Geometry check sheet. Reference: the model listing, model coordinates, mm. Coordinates: 2 decimals unless noted, no trailing zeros. Write each loop counter-clockwise with the first axis right and the second up, starting at its lowest first coordinate (ties: lowest second). Pieces come first, ordered by that corner, then holes. Notation, with made-up numbers: (7, 68.25) -> (28, 68.25) arc R14 cw to (28, 80.25) -> close; hole circle Ø9 at (68.25, -24). An arc over 180 degrees is marked (long way). Answer as CSV lines item,"result".
```python
from build123d import *

# Parameters (mm, degrees)
TD_SKETCH_R                             = 0.79248
TL_FEATURE_DEPTH                        = 21.0312
TDF_STD_SKETCH_W                        = 2.09296
TDF_STD_SKETCH_H                        = 2.09296
TDF_STD_FEATURE_DEPTH                   = 22.061040395
ISA_20_STD_FEATURE_DEPTH                = 22.061040395
ISA_20_STD_FEATURE_DEPTH_BACK           = 22.061040395
F_10BA_STD_FEATURE_DEPTH                = 22.061040395
F_10BA_STD_FEATURE_DEPTH_BACK           = 22.061040395
FRO_STD_FEATURE_DEPTH                   = 22.061040395
FRO_STD_FEATURE_DEPTH_BACK              = 22.061040395
C_STD_FEATURE_DEPTH                     = 22.061040395
C_STD_FEATURE_DEPTH_BACK                = 22.061040395
ERW_STD_FEATURE_DEPTH                   = 0.01905
H_STD_FEATURE_REACH                     = 22.955
H_STD_SKETCH_R                          = 0.01905
H_STD_SKETCH_3_R                        = 0.01905
FUNNEL_FINAL_DIAMETRE_STD_FEATURE_DEPTH = 2.499995
FUNNEL_FINAL_DIAMETRE_STD_FEATURE_DRAFT = -22.5
ROUND_BR_STD_FEATURE_START              = -1
ROUND_BR_STD_FEATURE_DEPTH              = 0.939082249


with BuildPart() as part:
    # TD_sketch → TL_feature (new body)
    with BuildSketch(Plane(origin=(0, 0, 0), x_dir=(1, 0, 0), z_dir=(0, 1, 0))):
        with Locations(Location((0, 0, 0), (0, 0, 270))):
            Circle(TD_SKETCH_R)
    extrude(amount=TL_FEATURE_DEPTH)

    # TDF_STD_sketch → TDF_STD_feature (cut, through all)
    with BuildSketch(Plane(origin=(0, 0, 0), x_dir=(1, 0, 0), z_dir=(0, 1, 0))):
        with Locations((-1.4224, 0)):
            Rectangle(TDF_STD_SKETCH_W, TDF_STD_SKETCH_H)
    extrude(amount=TDF_STD_FEATURE_DEPTH, mode=Mode.SUBTRACT)

    # ISA_20_STD_sketch → ISA_20_STD_feature (cut, two sides: drawn at the far end of the back side and taken through both)
    with BuildSketch(Plane(origin=(0, 0, 0), x_dir=(0, 0, -1), z_dir=(1, 0, 0)).offset(-ISA_20_STD_FEATURE_DEPTH_BACK)):
        Polygon((-12.955177728, 73.256388083), (-3.746467997, 21.0312), (-0.0381, 0), (0.0381, 0), (3.746467997, 21.0312), (12.955177728, 73.256388083), (12.955177728, -32.805303497), (-12.955177728, -32.805303497), align=None)
    extrude(amount=ISA_20_STD_FEATURE_DEPTH + ISA_20_STD_FEATURE_DEPTH_BACK, mode=Mode.SUBTRACT)

    # 10BA_STD_sketch → 10BA_STD_feature (cut, two sides: drawn at the far end of the back side and taken through both)
    with BuildSketch(Plane.XY.offset(-F_10BA_STD_FEATURE_DEPTH_BACK)):
        Polygon((-53.187771959, 0), (-0.37592, 0), (-0.29972, 0), (-0.091356515, 0.029283578), (3.611847997, 21.0312), (12.782529849, 73.04072126), (91.167207296, 2.243763904), (25.196905488, -70.796957355), align=None)
    extrude(amount=F_10BA_STD_FEATURE_DEPTH + F_10BA_STD_FEATURE_DEPTH_BACK, mode=Mode.SUBTRACT)

    # FRO_STD_sketch → FRO_STD_feature (cut, two sides: drawn at the far end of the back side and taken through both)
    with BuildSketch(Plane.XY.offset(-FRO_STD_FEATURE_DEPTH_BACK)):
        with BuildLine():
            Line((-0.37592, 52.149873762), (-0.37592, 0.0254))
            ThreePointArc((-0.37592, 0.0254), (-0.368480512, 0.007439488), (-0.35052, 0))
            Line((-0.35052, 0), (51.773953762, 0))
            Line((51.773953762, 0), (-21.941183964, -73.715137726))
            Line((-21.941183964, -73.715137726), (-74.091057726, -21.565263964))
            Line((-74.091057726, -21.565263964), (-0.37592, 52.149873762))
        make_face()
    extrude(amount=FRO_STD_FEATURE_DEPTH + FRO_STD_FEATURE_DEPTH_BACK, mode=Mode.SUBTRACT)

    # C_STD_sketch → C_STD_feature (cut, two sides: drawn at the far end of the back side and taken through both)
    with BuildSketch(Plane(origin=(0, 0, 0), x_dir=(0, 0, -1), z_dir=(1, 0, 0)).offset(-C_STD_FEATURE_DEPTH_BACK)):
        with BuildLine():
            Line((-51.36762506, -8.882670253), (-0.03551364, 0))
            ThreePointArc((-0.03551364, 0), (0, 0.003050032), (0.03551364, 0))
            Line((0.03551364, 0), (51.36762506, -8.882670253))
            Line((51.36762506, -8.882670253), (51.36762506, -113.072640858))
            Line((51.36762506, -113.072640858), (-51.36762506, -113.072640858))
            Line((-51.36762506, -113.072640858), (-51.36762506, -8.882670253))
        make_face()
    extrude(amount=C_STD_FEATURE_DEPTH + C_STD_FEATURE_DEPTH_BACK, mode=Mode.SUBTRACT)


with BuildPart() as body_2:
    # ERW_STD_sketch → ERW_STD_feature (new, symmetric)
    with BuildSketch(Plane.XY):
        Polygon((-0.182120032, 0.06096), (-0.182120032, 0), (-0.321820032, 0), (-0.275883377, 0.06096), align=None)
    extrude(amount=ERW_STD_FEATURE_DEPTH, both=True)

    # H_STD_sketch → H_STD_feature (add, up to next)
    with BuildSketch(Plane(origin=(-0.096909952, 0.110156063, 0), x_dir=(0, 0, -1), z_dir=(0.8660254037844415, 0.4999999999999953, 0)), mode=Mode.PRIVATE) as h_std_feature_sk1:
        with Locations(Location((0, 0, 0), (0, 0, 90))):
            Circle(H_STD_SKETCH_R)
    h_std_feature_tool1 = extrude(h_std_feature_sk1.sketch, amount=-H_STD_FEATURE_REACH, mode=Mode.PRIVATE) - body_2.part
    add(h_std_feature_tool1.solids().sort_by_distance((-0.09691, 0.110156, 0))[0])


with BuildPart() as funnel_final_diametre_std_feature_tool:
    # H_STD_sketch<3> → funnel_final_diametre_STD_feature (with draft: the straight prism first)
    with BuildSketch(Plane(origin=(-0.096909952, 0.110156063, 0), x_dir=(0, 0, -1), z_dir=(0.8660254037844415, 0.4999999999999953, 0))):
        with Locations(Location((0, 0, 0), (0, 0, 90))):
            Circle(H_STD_SKETCH_3_R)
    extrude(amount=FUNNEL_FINAL_DIAMETRE_STD_FEATURE_DEPTH)
    # funnel_final_diametre_STD_feature: the draft: its side faces are tilted about the plane it starts from
    funnel_final_diametre_std_feature_sides = [funnel_final_diametre_std_feature_tool.faces().sort_by_distance(p)[0] for p in [
        (0.995144638, 0.718657029, 0),
    ]]
    draft(funnel_final_diametre_std_feature_sides, Plane(origin=(-0.096909952, 0.110156063, 0), x_dir=(0, 0, -1), z_dir=(0.8660254037844415, 0.4999999999999953, 0)), FUNNEL_FINAL_DIAMETRE_STD_FEATURE_DRAFT)


with BuildPart() as body_2_1:
    add(body_2.part)

    # funnel_final_diametre_STD_feature: add funnel_final_diametre_std_feature_tool
    add(funnel_final_diametre_std_feature_tool.part)

    # ROUND_BR_STD_feature: read off the stored shape, not the designer's step
    # ROUND_BR_STD_feature outline → ROUND_BR_STD_feature (cut)
    with BuildSketch(Plane(origin=(0, 0, 0), x_dir=(0.79863551004729, -0.601815023152052, 0), z_dir=(0.601815023152052, 0.79863551004729, 0)).offset(ROUND_BR_STD_FEATURE_START)):
        with BuildLine():
            Line((-0.257016905, -0.01905), (-0.237966905, -0.01905))
            ThreePointArc((-0.237966905, -0.01905), (-0.251437289, -0.013470384), (-0.257016905, 0))
            Line((-0.257016905, 0), (-0.257016905, -0.01905))
        make_face()
        with BuildLine():
            Line((-0.257016905, 0.01905), (-0.257016905, 0))
            ThreePointArc((-0.257016905, 0), (-0.251437289, 0.013470384), (-0.237966905, 0.01905))
            Line((-0.237966905, 0.01905), (-0.257016905, 0.01905))
        make_face()
    extrude(amount=ROUND_BR_STD_FEATURE_DEPTH, mode=Mode.SUBTRACT)


with BuildPart() as part_1:
    add(part.part)

    # COMBINE_STD_feature: cut body 2
    add(body_2_1.part, mode=Mode.SUBTRACT)


solid = part_1.part
```
Item 1: Thickness scan on probe 1 along Z at (x, y) = (0.3, 19.75); probe 2 along X at (y, z) = (13.5, 0.05); probe 3 along X at (y, z) = (5.5, 0.4). Record the ranges inside material, lowest first.
Responses:
probe 1,"z = -0.73 to 0.73"
probe 2,"x = -0.38 to 0.79"
probe 3,"x = -0.38 to 0.68"
Item 2: Cross-section at B-B, the plane z = -0.4. Record the cut outline in (x, y).
Responses:
outline,"(-0.38, 2.05) -> (0.27, 2.05) -> (0.68, 4.43) -> (0.68, 21.03) -> (-0.38, 21.03) -> close"
Item 3: Cross-section at A-A, the plane y = 15.75. Record the cut outline in (x, z), plus the area to 3 significant figures.
Responses:
outline,"(-0.38, -0.7) arc R0.79 ccw (long way) to (-0.38, 0.7) -> close"
area,"1.56 mm2"
Item 4: Cross-section at C-C, the plane x = 0.2. Record the cut outline in (y, z), plus the area to 3 significant figures.
Responses:
outline,"(1.68, -0.33) -> (4.13, -0.77) -> (21.03, -0.77) -> (21.03, 0.77) -> (4.13, 0.77) -> (1.68, 0.33) -> close"
area,"28.6 mm2"
